Work out the finished part from the listing and answer in its coordinate system (mm). Coordinates: 2 decimals unless noted, no trailing zeros. Loops run counter-clockwise (first coordinate to the right, second up) from the corner with the lowest first, then second, coordinate; pieces in that order, holes last. Notation, with made-up numbers: (33, 56) - (89, 56) arc R7 cw to (89, 62) - close; hole circle Ø3 at (19, -17). An arc over 180 degrees is marked (long way). Write each question's results on one line, items separated by ' | '. Start each with the question number.
Item 1: Section C-C, the plane z = 3.1 is taken. Write down the section's boundary in (x, y).
Item 2: Section A-A, the plane y = 0 is taken. Write down the section's boundary in (x, z).
Item 3: Consider probe 1 along Y at (x, z) = (0, 0.85); probe 2 along Y at (x, z) = (-0.25, 1.8); probe 3 along X at (y, z) = (-1.75, 1.75). Determine where each line is inside the solid, lowest interval first. Write a range as [from, to].
Item 4: Each of these flat-tipped pins is pushed along its axis until it touches: pin 1 Ø4 at (x, y) = (-3, 4) entering from +Z; pin 2 Ø1 at (x, z) = (-4.5, 1) entering from -Y; pin 3 Ø1.5 at (x, z) = (-3, 0.5) entering from -Y; pin 4 Ø4 at (x, y) = (0, 0) entering from +Z. Where does it stop, or does it pass through?
Item 5: Section D-D, the plane z = 0.3 is taken. Write down the section's boundary in (x, y).
Item 6: For a pull along Y with two mould halves and no side action, classify faces 1 (the face through (2, -2, 0)), 2 (the face through (-0.6, -2.7, 3.38)), 3 (the face through (2.003, 0.631, 1.774)) as +Y half, -Y half, draft (parallel to the pull), parting line (faces both ways), or undercut.
from build123d import *

# Parameters (mm, degrees)
SKETCH1_R                   = 8
BOSS_EXTRUDE1_DEPTH         = 3.5
CHAMFER1_SIZE               = 2.5
CHAMFER1_SIZE2              = 5.5
TAP_DRILL_FOR_M5X0_8_TAP1_D = 4.2


with BuildPart() as part:
    # Sketch1 → Boss-Extrude1 (new body)
    with BuildSketch(Plane.XY):
        Circle(SKETCH1_R)
    extrude(amount=BOSS_EXTRUDE1_DEPTH)

    # Chamfer1
    chamfer1_edges = [part.edges().sort_by_distance(p)[0] for p in [
        (-8, 0, 3.5),
    ]]
    chamfer1_side = [part.faces().sort_by_distance(p)[0] for p in [
        (-8, 0, 1.75),
    ]]
    chamfer(chamfer1_edges, length=CHAMFER1_SIZE, length2=CHAMFER1_SIZE2, reference=chamfer1_side[0])

    # Tap Drill for M5x0.8 Tap1 (through all)
    with Locations(Plane(origin=(0, 0, 0), x_dir=(-1, 0, 0), z_dir=(0, 0, -1))):
        with Locations((0, 0)):
            Hole(TAP_DRILL_FOR_M5X0_8_TAP1_D / 2)


solid = part.part
Answer key:
1) outline: circle Ø6.76 at (0, 0); hole circle Ø4.2 at (0, 0)
2) outline: (-8, 0) - (-2.1, 0) - (-2.1, 3.5) - (-2.5, 3.5) - (-8, 1) - close; (2.1, 0) - (8, 0) - (8, 1) - (2.5, 3.5) - (2.1, 3.5) - close
3) probe 1: y = [-8, -2.1], [2.1, 8] | probe 2: y = [-6.23, -2.09], [2.09, 6.23] | probe 3: x = [-6.1, -1.16], [1.16, 6.1]
4) pin 1: stops at z = 3.27 | pin 2: stops at y = -6.93 | pin 3: stops at y = -7.68 | pin 4: passes through
5) outline: circle Ø16 at (0, 0); hole circle Ø4.2 at (0, 0)
6) face 1: draft | face 2: parting line | face 3: undercut
